Source: CAD feature listing. Evaluate the final solid. Frame: model axes, mm. Give positions to 0.01 mm unless a question says otherwise; leave off trailing zeros. Order: outer loops, then holes, each group sorted by start corner. A loop starts at its lowest first (then second) coordinate and runs counter-clockwise, first axis right, second up. Notation, with made-up numbers: M -18,24 L 18,24 A10 cw 18,38 Z; hole C 1.25,55 d9. An arc over 180 degrees is marked long. Use CSV: the item, a comma, the result in double quotes. Start each with the question number.
Item 1: Section query B-B on y = -114.5. Return loops of the section in (x, z) (3 decimals).
Item 2: Section query C-C on y = 17.68. Return loops of the section in (x, z).
Item 3: First-contact query: pin 1 (8.5 mm diameter, centred on y = -17.68, z = -17.68, fed in from -X); pin 2 (7.5 mm diameter, centred on y = 17.68, z = -17.68, fed in from +X); pin 3 (5.5 mm diameter, centred on y = -114.5, z = 17.68, fed in from -X). Flat tips, straight axial feed; report the tip coordinate or a pass-through.
Item 4: Section query A-A on z = 17.68. Return loops of the section in (x, y) (3 decimals), and give its area (3 significant figures).
Item 5: Ray query, probe 1 along Z at (x, y) = (6.5, -114.5); probe 2 along Y at (x, z) = (1.8, -17.68) (3 decimals); probe 3 along Y at (x, z) = (9, 17.68). Return the intervals inside material, ascending. Write a range as from..to.
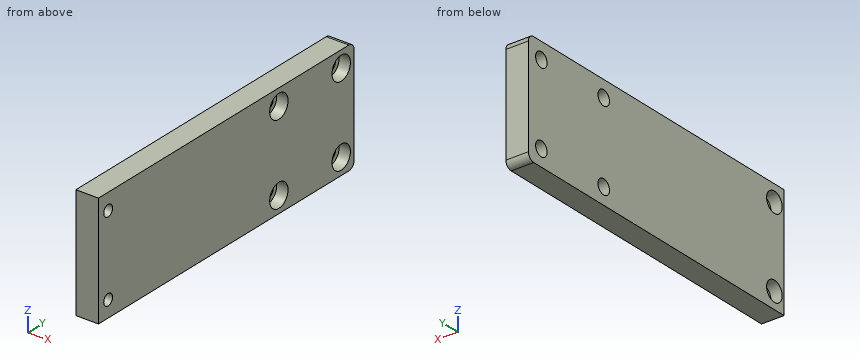
from build123d import *

# Parameters (mm, degrees)
CROQUIS1_R              = 3.25
CROQUIS1_R_2            = 2.5
SALIENTE_EXTRUIR1_DEPTH = 10
CROQUIS5_R              = 5.2
CORTAR_EXTRUIR2_DEPTH   = 5
FILLET1_R               = 3
SKETCH1_R               = 4.425
CUT_EXTRUDE1_DEPTH      = 5


with BuildPart() as part:
    # Croquis1 → Saliente-Extruir1 (new body)
    with BuildSketch(Plane(origin=(0, 0, 0), x_dir=(0, 0, -1), z_dir=(1, 0, 0))):
        Polygon((-25, -120), (25, -120), (25, 25), (0, 25), (-25, 25), (-25, 0), align=None)
        with Locations((-17.68, 17.68)):
            Circle(CROQUIS1_R, mode=Mode.SUBTRACT)
        with Locations(Location((17.68, 17.68, 0), (0, 0, 180))):
            Circle(CROQUIS1_R, mode=Mode.SUBTRACT)
        with Locations((17.68, -17.68)):
            Circle(CROQUIS1_R, mode=Mode.SUBTRACT)
        with Locations(Location((-17.68, -17.68, 0), (0, 0, 180))):
            Circle(CROQUIS1_R, mode=Mode.SUBTRACT)
        with Locations((-17.68, -114.5)):
            Circle(CROQUIS1_R_2, mode=Mode.SUBTRACT)
        with Locations(Location((17.68, -114.5, 0), (0, 0, 180))):
            Circle(CROQUIS1_R_2, mode=Mode.SUBTRACT)
    extrude(amount=SALIENTE_EXTRUIR1_DEPTH)

    # Croquis5 → Cortar-Extruir2 (cut)
    with BuildSketch(Plane(origin=(10, 0, 0), x_dir=(0, 0, -1), z_dir=(1, 0, 0))):
        with Locations((17.68, 17.68)):
            Circle(CROQUIS5_R)
        with Locations((-17.68, 17.68)):
            Circle(CROQUIS5_R)
        with Locations((-17.68, -17.68)):
            Circle(CROQUIS5_R)
        with Locations((17.68, -17.68)):
            Circle(CROQUIS5_R)
    extrude(amount=-CORTAR_EXTRUIR2_DEPTH, mode=Mode.SUBTRACT)

    # Fillet1
    fillet1_edges = [part.edges().sort_by_distance(p)[0] for p in [
        (5, 25, -25),
        (5, 25, 25),
    ]]
    fillet(fillet1_edges, radius=FILLET1_R)

    # Sketch1 → Cut-Extrude1 (cut)
    with BuildSketch(Plane.ZY):
        with Locations((17.68, -114.5)):
            Circle(SKETCH1_R)
        with Locations(Location((-17.68, -114.5, 0), (0, 0, 180))):
            Circle(SKETCH1_R)
    extrude(amount=-CUT_EXTRUDE1_DEPTH, mode=Mode.SUBTRACT)


solid = part.part
Verdict:
1,outline,"M 0,-25 L 10,-25 L 10,-20.18 L 5,-20.18 L 5,-22.105 L 0,-22.105 Z; M 0,-13.255 L 5,-13.255 L 5,-15.18 L 10,-15.18 L 10,15.18 L 5,15.18 L 5,13.255 L 0,13.255 Z; M 0,22.105 L 5,22.105 L 5,20.18 L 10,20.18 L 10,25 L 0,25 Z"
2,outline,"M 0,-25 L 10,-25 L 10,-22.88 L 5,-22.88 L 5,-20.93 L 0,-20.93 Z; M 0,-14.43 L 5,-14.43 L 5,-12.48 L 10,-12.48 L 10,12.48 L 5,12.48 L 5,14.43 L 0,14.43 Z; M 0,20.93 L 5,20.93 L 5,22.88 L 10,22.88 L 10,25 L 0,25 Z"
3,pin 1,"x = 0"
3,pin 2,"x = 5"
3,pin 3,"x = 5"
4,outline,"M 0,-120 L 10,-120 L 10,-117 L 5,-117 L 5,-118.925 L 0,-118.925 Z; M 0,-110.075 L 5,-110.075 L 5,-112 L 10,-112 L 10,-22.88 L 5,-22.88 L 5,-20.93 L 0,-20.93 Z; M 0,-14.43 L 5,-14.43 L 5,-12.48 L 10,-12.48 L 10,12.48 L 5,12.48 L 5,14.43 L 0,14.43 Z; M 0,20.93 L 5,20.93 L 5,22.88 L 10,22.88 L 10,25 L 0,25 Z"
4,area,"1,210 mm2"
5,probe 1,"-25..-20.18, -15.18..15.18, 20.18..25"
5,probe 2,"-120..-118.925, -110.075..-20.93, -14.43..14.43, 20.93..25"
5,probe 3,"-120..-117, -112..-22.88, -12.48..12.48, 22.88..25"
